Read the model definition and answer for the solid it produces. Units are mm, in the model's axes. Face numbers are marked on the shaded views. A direction names the side the tool comes from. Round coordinates to 2 decimals unless told otherwise and drop trailing zeros. Loops run counter-clockwise (first coordinate to the right, second up) from the corner with the lowest first, then second, coordinate; pieces in that order, holes last. Notation, with made-up numbers: (6.25, 72) -> (20.25, 72) arc R18 cw to (20.25, 96) -> close; hole circle Ø2 at (54, -25.5). An arc over 180 degrees is marked (long way). Put each result on its own line as item: value.
from build123d import *

# Parameters (mm, degrees)
BOSS_EXTRUDE1_DEPTH  = 30
SKETCH4_W            = 35
SKETCH4_H            = 61.907073604
BOSS_EXTRUDE2_DEPTH  = 10
SKETCH5_W            = 23.104058428
SKETCH5_H            = 61.907073604
BOSS_EXTRUDE3_DEPTH  = 10
SKETCH6_W            = 11.552029214
SKETCH6_H            = 61.907073604
BOSS_EXTRUDE5_DEPTH  = 8
SKETCH8_W            = 11.895941572
SKETCH8_H            = 11.490805908
SKETCH8_H_2          = 11.569660377
BOSS_EXTRUDE6_DEPTH  = 2
SKETCH9_W            = 11.552029214
SKETCH9_H            = 11.763067294
SKETCH9_H_2          = 11.444663326
BOSS_EXTRUDE7_DEPTH  = 2
SKETCH10_W           = 11.552029214
SKETCH10_H           = 12.016051613
SKETCH10_H_2         = 11.413040286
BOSS_EXTRUDE8_DEPTH  = 2.5
SKETCH11_W           = 64.341621443
SKETCH11_H           = 28.817099519
BOSS_EXTRUDE9_DEPTH  = 10
SKETCH12_W           = 64.341621443
SKETCH12_H           = 19.413143898
BOSS_EXTRUDE10_DEPTH = 10
SKETCH13_W           = 64.341621443
SKETCH13_H           = 10.936081157
BOSS_EXTRUDE11_DEPTH = 8
SKETCH14_W           = 7
SKETCH14_H           = 9.302294552
BOSS_EXTRUDE12_DEPTH = 2
SKETCH15_W           = 6.954726323
SKETCH15_H           = 8.57872381
SKETCH15_W_2         = 6.927384131
BOSS_EXTRUDE13_DEPTH = 2
SKETCH16_W           = 6.926390046
SKETCH16_H           = 10.936081157
SKETCH16_W_2         = 6.728901939
BOSS_EXTRUDE14_DEPTH = 2
SKETCH17_W           = 58.417259869
SKETCH17_H           = 32.138328606
BOSS_EXTRUDE15_DEPTH = 10
SKETCH18_W           = 58.429148121
SKETCH18_H           = 22.541723998
BOSS_EXTRUDE16_DEPTH = 10
SKETCH19_W           = 58.429148121
SKETCH19_H           = 12.314239644
BOSS_EXTRUDE17_DEPTH = 8
SKETCH20_W           = 30
SKETCH20_H           = 115.814918598
BOSS_EXTRUDE18_DEPTH = 25
SKETCH21_W           = 6.015404917
SKETCH21_H           = 9.543718354
SKETCH21_W_2         = 6.015404916
BOSS_EXTRUDE19_DEPTH = 2
SKETCH22_W           = 6.058740194
SKETCH22_H           = 10.280370608
SKETCH22_W_2         = 6.028288377
BOSS_EXTRUDE20_DEPTH = 2
SKETCH23_W           = 6.002521456
SKETCH23_H           = 12.314239644
SKETCH23_W_2         = 6.105589141
BOSS_EXTRUDE21_DEPTH = 2
CUT_EXTRUDE2_DEPTH   = 28


with BuildPart() as part:
    # Sketch1 → Boss-Extrude1 (new body)
    with BuildSketch(Plane.XY):
        with BuildLine():
            Line((-237.128848942, 435.351344416), (-237.128848942, 421.091849934))
            Line((-237.128848942, 421.091849934), (-206.17531214, 421.091849934))
            Line((-206.17531214, 421.091849934), (-206.17531214, 408.223525645))
            Line((-206.17531214, 408.223525645), (-160.266695759, 408.223525645))
            Line((-160.266695759, 408.223525645), (-160.266695759, 395.355201356))
            Line((-160.266695759, 395.355201356), (-131.052121698, 395.355201356))
            Line((-131.052121698, 395.355201356), (-101.837547638, 395.355201356))
            Line((-101.837547638, 395.355201356), (-95.925074316, 395.355201356))
            Line((-95.925074316, 395.355201356), (-95.925074316, 379.704536681))
            Line((-95.925074316, 379.704536681), (-82.013372382, 379.704536681))
            Line((-82.013372382, 379.704536681), (-82.013372382, 356.75022849))
            Line((-82.013372382, 356.75022849), (-22.540846616, 356.75022849))
            Line((-22.540846616, 356.75022849), (-22.540846616, 379.704536681))
            Line((-22.540846616, 379.704536681), (-8.629144682, 379.704536681))
            Line((-8.629144682, 379.704536681), (-8.629144682, 395.355201356))
            Line((-8.629144682, 395.355201356), (0, 395.355201356))
            Line((0, 395.355201356), (0, 414.657687789))
            ThreePointArc((0, 414.657687789), (40.25698747, 454.91467526), (0, 495.17166273))
            Line((0, 495.17166273), (0, 516.734800727))
            Line((0, 516.734800727), (-8.629144682, 516.734800727))
            Line((-8.629144682, 516.734800727), (-8.629144682, 529.255332468))
            Line((-8.629144682, 529.255332468), (-22.540846616, 529.255332468))
            Line((-22.540846616, 529.255332468), (-22.540846616, 551.86184811))
            Line((-22.540846616, 551.86184811), (-82.013372382, 551.86184811))
            Line((-82.013372382, 551.86184811), (-82.013372382, 527.168577178))
            Line((-82.013372382, 527.168577178), (-95.925074316, 527.168577178))
            Line((-95.925074316, 527.168577178), (-95.925074316, 513.256875244))
            Line((-95.925074316, 513.256875244), (-101.837547638, 513.256875244))
            Line((-101.837547638, 513.256875244), (-101.837547638, 511.170119954))
            Line((-101.837547638, 511.170119954), (-131.052121698, 511.170119954))
            Line((-131.052121698, 511.170119954), (-160.266695759, 511.170119954))
            Line((-160.266695759, 511.170119954), (-160.266695759, 495.17166273))
            Line((-160.266695759, 495.17166273), (-206.17531214, 492.737114892))
            Line((-206.17531214, 492.737114892), (-206.17531214, 482.998923538))
            Line((-206.17531214, 482.998923538), (-237.128848942, 482.998923538))
            Line((-237.128848942, 482.998923538), (-237.128848942, 464.565918476))
            Line((-237.128848942, 464.565918476), (-237.128848942, 454.132142026))
            Line((-237.128848942, 454.132142026), (-237.128848942, 435.351344416))
        make_face()
    extrude(amount=BOSS_EXTRUDE1_DEPTH)

    # Sketch4 → Boss-Extrude2 (add)
    with BuildSketch(Plane(origin=(0, 0, 0), x_dir=(-1, 0, 0), z_dir=(0, 0, -1))):
        with Locations((254.628848942, 452.045386736)):
            Rectangle(SKETCH4_W, SKETCH4_H)
    extrude(amount=-BOSS_EXTRUDE2_DEPTH)

    # Sketch5 → Boss-Extrude3 (add)
    with BuildSketch(Plane.XY.offset(10)):
        with Locations((-248.680878156, 452.045386736)):
            Rectangle(SKETCH5_W, SKETCH5_H)
    extrude(amount=BOSS_EXTRUDE3_DEPTH)

    # Sketch6 → Boss-Extrude5 (add)
    with BuildSketch(Plane.XY.offset(20)):
        with Locations((-242.904863549, 452.045386736)):
            Rectangle(SKETCH6_W, SKETCH6_H)
    extrude(amount=BOSS_EXTRUDE5_DEPTH)

    # Sketch8 → Boss-Extrude6 (add)
    with BuildSketch(Plane.XY.offset(10)):
        with Locations((-266.180878156, 425.34644698)):
            Rectangle(SKETCH8_W, SKETCH8_H)
        with Locations((-266.180878156, 478.783753727)):
            Rectangle(SKETCH8_W, SKETCH8_H_2)
    extrude(amount=BOSS_EXTRUDE6_DEPTH)

    # Sketch9 → Boss-Extrude7 (add)
    with BuildSketch(Plane.XY.offset(20)):
        with Locations((-254.456892763, 478.687050268)):
            Rectangle(SKETCH9_W, SKETCH9_H)
        with Locations((-254.456892763, 425.369518271)):
            Rectangle(SKETCH9_W, SKETCH9_H_2)
    extrude(amount=BOSS_EXTRUDE7_DEPTH)

    # Sketch10 → Boss-Extrude8 (add)
    with BuildSketch(Plane.XY.offset(28)):
        with Locations((-242.904863549, 478.560558109)):
            Rectangle(SKETCH10_W, SKETCH10_H)
        with Locations((-242.904863549, 425.385329791)):
            Rectangle(SKETCH10_W, SKETCH10_H_2)
    extrude(amount=BOSS_EXTRUDE8_DEPTH)

    # Sketch11 → Boss-Extrude9 (add)
    with BuildSketch(Plane(origin=(0, 0, 0), x_dir=(-1, 0, 0), z_dir=(0, 0, -1))):
        with Locations((128.095885038, 380.946651597)):
            Rectangle(SKETCH11_W, SKETCH11_H)
    extrude(amount=-BOSS_EXTRUDE9_DEPTH)

    # Sketch12 → Boss-Extrude10 (add)
    with BuildSketch(Plane.XY.offset(10)):
        with Locations((-128.095885038, 385.648629407)):
            Rectangle(SKETCH12_W, SKETCH12_H)
    extrude(amount=BOSS_EXTRUDE10_DEPTH)

    # Sketch13 → Boss-Extrude11 (add)
    with BuildSketch(Plane.XY.offset(20)):
        with Locations((-128.095885038, 389.887160778)):
            Rectangle(SKETCH13_W, SKETCH13_H)
    extrude(amount=BOSS_EXTRUDE11_DEPTH)

    # Sketch14 → Boss-Extrude12 (add)
    with BuildSketch(Plane.XY.offset(10)):
        with Locations((-157.909862062, 371.189249113)):
            Rectangle(SKETCH14_W, SKETCH14_H)
        with Locations((-98.195021783, 371.189249113)):
            Rectangle(SKETCH14_W, SKETCH14_H)
    extrude(amount=BOSS_EXTRUDE12_DEPTH)

    # Sketch15 → Boss-Extrude13 (add)
    with BuildSketch(Plane.XY.offset(20)):
        with Locations((-157.932498901, 380.129758294)):
            Rectangle(SKETCH15_W, SKETCH15_H)
        with Locations((-98.158713849, 380.129758294)):
            Rectangle(SKETCH15_W_2, SKETCH15_H)
    extrude(amount=BOSS_EXTRUDE13_DEPTH)

    # Sketch16 → Boss-Extrude14 (add)
    with BuildSketch(Plane.XY.offset(28)):
        with Locations((-157.946667039, 389.887160778)):
            Rectangle(SKETCH16_W, SKETCH16_H)
        with Locations((-98.257954944, 389.887160778)):
            Rectangle(SKETCH16_W_2, SKETCH16_H)
    extrude(amount=BOSS_EXTRUDE14_DEPTH)

    # Sketch17 → Boss-Extrude15 (add)
    with BuildSketch(Plane(origin=(0, 0, 0), x_dir=(-1, 0, 0), z_dir=(0, 0, -1))):
        with Locations((131.046177572, 527.239284257)):
            Rectangle(SKETCH17_W, SKETCH17_H)
    extrude(amount=-BOSS_EXTRUDE15_DEPTH)

    # Sketch18 → Boss-Extrude16 (add)
    with BuildSketch(Plane.XY.offset(10)):
        with Locations((-131.052121699, 522.440981953)):
            Rectangle(SKETCH18_W, SKETCH18_H)
    extrude(amount=BOSS_EXTRUDE16_DEPTH)

    # Sketch19 → Boss-Extrude17 (add)
    with BuildSketch(Plane.XY.offset(20)):
        with Locations((-131.052121699, 517.327239776)):
            Rectangle(SKETCH19_W, SKETCH19_H)
    extrude(amount=BOSS_EXTRUDE17_DEPTH)

    # Sketch20 → Boss-Extrude18 (add)
    with BuildSketch(Plane.ZY.offset(206.17531214)):
        with Locations((15, 453.262660655)):
            Rectangle(SKETCH20_W, SKETCH20_H)
    extrude(amount=BOSS_EXTRUDE18_DEPTH)

    # Sketch21 → Boss-Extrude19 (add)
    with BuildSketch(Plane.XY.offset(10)):
        with Locations((-158.254585418, 538.536589383)):
            Rectangle(SKETCH21_W, SKETCH21_H)
        with Locations((-103.834847481, 538.536589383)):
            Rectangle(SKETCH21_W_2, SKETCH21_H)
    extrude(amount=BOSS_EXTRUDE19_DEPTH)

    # Sketch22 → Boss-Extrude20 (add)
    with BuildSketch(Plane.XY.offset(20)):
        with Locations((-158.232917779, 528.624544902)):
            Rectangle(SKETCH22_W, SKETCH22_H)
        with Locations((-103.828405751, 528.624544902)):
            Rectangle(SKETCH22_W_2, SKETCH22_H)
    extrude(amount=BOSS_EXTRUDE20_DEPTH)

    # Sketch23 → Boss-Extrude21 (add)
    with BuildSketch(Plane.XY.offset(28)):
        with Locations((-158.261027148, 517.327239776)):
            Rectangle(SKETCH23_W, SKETCH23_H)
        with Locations((-103.789755369, 517.327239776)):
            Rectangle(SKETCH23_W_2, SKETCH23_H)
    extrude(amount=BOSS_EXTRUDE21_DEPTH)

    # Sketch24 → Cut-Extrude2 (cut)
    with BuildSketch(Plane(origin=(0, 0, 0), x_dir=(-1, 0, 0), z_dir=(0, 0, -1))):
        with BuildLine():
            Line((228.979940095, 479.759783132), (228.979940095, 506.732020696))
            Line((228.979940095, 506.732020696), (209.499990744, 506.732020696))
            Line((209.499990744, 506.732020696), (209.499990744, 490.248986629))
            Line((209.499990744, 490.248986629), (156.454590203, 490.248986629))
            Line((156.454590203, 490.248986629), (156.454590203, 511.227393623))
            Line((156.454590203, 511.227393623), (107.005488005, 511.227393623))
            Line((107.005488005, 511.227393623), (92.919986166, 511.227393623))
            Line((92.919986166, 511.227393623), (92.919986166, 524.863358168))
            Line((92.919986166, 524.863358168), (77.935409742, 524.863358168))
            Line((77.935409742, 524.863358168), (77.935409742, 546.890685512))
            Line((77.935409742, 546.890685512), (26.088775316, 546.890685512))
            Line((26.088775316, 546.890685512), (26.088775316, 527.710427689))
            Line((26.088775316, 527.710427689), (13.202039591, 527.710427689))
            Line((13.202039591, 527.710427689), (13.202039591, 514.374154672))
            Line((13.202039591, 514.374154672), (4.510985265, 514.374154672))
            Line((4.510985265, 514.374154672), (4.510985265, 493.245901914))
            ThreePointArc((4.510985265, 493.245901914), (-34.748604966, 456.383843911), (2.113453037, 417.124253681))
            Line((2.113453037, 417.124253681), (2.113453037, 396.745229744))
            Line((2.113453037, 396.745229744), (10.804507363, 396.745229744))
            Line((10.804507363, 396.745229744), (10.804507363, 381.161270263))
            Line((10.804507363, 381.161270263), (26.088775316, 381.161270263))
            Line((26.088775316, 381.161270263), (26.088775316, 358.684405627))
            Line((26.088775316, 358.684405627), (80.632633499, 358.684405627))
            Line((80.632633499, 358.684405627), (80.632633499, 381.161270263))
            Line((80.632633499, 381.161270263), (80.632633499, 390.751399175))
            Line((80.632633499, 390.751399175), (80.632633499, 399.4424535))
            Line((80.632633499, 399.4424535), (156.454590203, 399.4424535))
            Line((156.454590203, 399.4424535), (156.454590203, 410.531040054))
            Line((156.454590203, 410.531040054), (209.499990744, 410.531040054))
            Line((209.499990744, 410.531040054), (209.499990744, 399.4424535))
            Line((209.499990744, 399.4424535), (228.979940095, 399.4424535))
            Line((228.979940095, 399.4424535), (228.979940095, 424.017158836))
            Line((228.979940095, 424.017158836), (228.979940095, 479.759783132))
        make_face()
    extrude(amount=-CUT_EXTRUDE2_DEPTH, mode=Mode.SUBTRACT)


solid = part.part
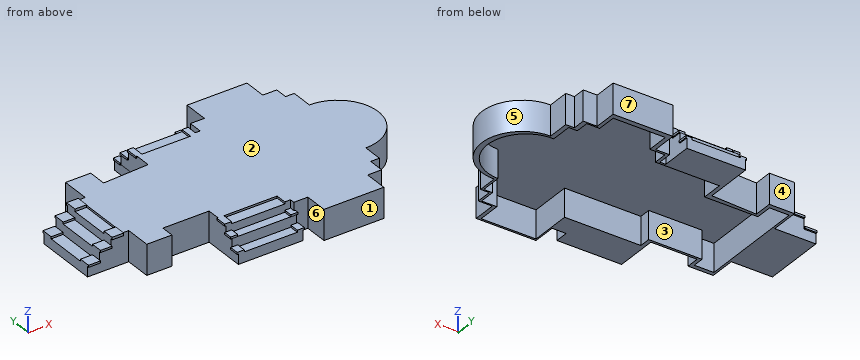
Item 1: Which of the six approach directions +Z, -Z, +X, -X, +Y, -Y give full straight-line access (tool end or side, diameter ignored) to the marked faces 1, 2, 3 and 4?
Derived:
face 1: +Z, -Z, +X, -X, -Y
face 2: +Z, +X, +Y, -Y
face 3: -Z
face 4: +Z, -Z, -X, +Y
Item 2: Flat-ended cylindrical pins translate along their axes: pin 1 Ø10 at (y, z) = (394.5, 19) entering from +X; pin 2 Ø2 at (x, y) = (-132.5, 517.5) entering from -Z; pin 3 Ø2 at (y, z) = (424, 29) entering from +X; pin 4 Ø1.6 at (x, z) = (-254.5, 20.5) entering from +Y. Find the tip coordinate at first contact, or state that the pin passes through.
Derived:
pin 1: stops at x = 0
pin 2: stops at z = 0
pin 3: stops at x = 26.94
pin 4: stops at y = 484.57
Item 3: The part is cut by section A-A (x = -219.5). Determine the outline of the cut face in (y, z).
Derived:
outline: (395.36, 0) -> (399.44, 0) -> (399.44, 28) -> (506.73, 28) -> (506.73, 0) -> (511.17, 0) -> (511.17, 30) -> (395.36, 30) -> close
Item 4: The part is cut by section B-B (y = 461). Determine the outline of the cut face in (x, z).
Derived:
outline: (-272.13, 0) -> (-228.98, 0) -> (-228.98, 28) -> (34.32, 28) -> (34.32, 0) -> (39.79, 0) -> (39.79, 30) -> (-237.13, 30) -> (-237.13, 28) -> (-248.68, 28) -> (-248.68, 20) -> (-260.23, 20) -> (-260.23, 10) -> (-272.13, 10) -> close
Item 5: The part is cut by section C-C (x = -35.5). Determine the outline of the cut face in (y, z).
Derived:
outline: (356.75, 0) -> (358.68, 0) -> (358.68, 28) -> (546.89, 28) -> (546.89, 0) -> (551.86, 0) -> (551.86, 30) -> (356.75, 30) -> close
Item 6: For a pull along X with two mould halves and no side action, classify the marked faces 5, 6 and 7 as pulls with the +X half, pulls with the -X half, needs draft (parallel to the pull), parting line crosses it, or undercut.
Derived:
face 5: pulls with the +X half
face 6: undercut
face 7: needs draft
Item 7: Find the intervals of material crossed by line 1 along X through (y, z) = (367.5, 3); line 2 along X through (y, z) = (400, 10.5); line 3 along Y through (x, z) = (-43, 5.5), in increasing order.
Derived:
line 1: x = -160.27 to -95.93, -82.01 to -80.63, -26.09 to -22.54
line 2: x = -231.18 to -228.98, -209.5 to -206.18, -160.27 to -156.45, -2.11 to 0
line 3: y = 356.75 to 358.68, 546.89 to 551.86
